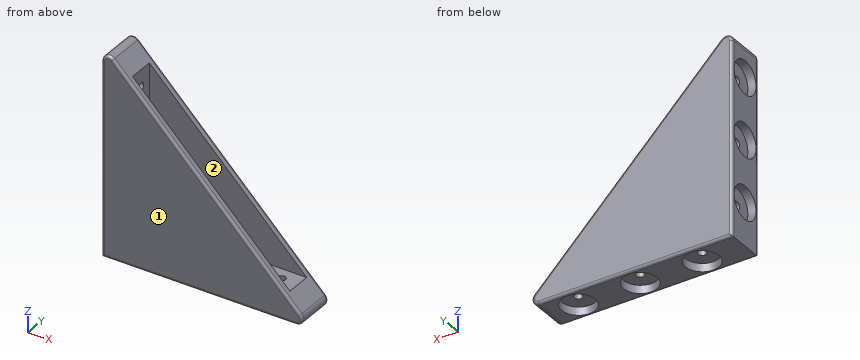
from build123d import *

# Parameters (mm, degrees)
F1_DEPTH  = 7.5
F2_R      = 6.375
F3_DEPTH  = 3.125
F4_R      = 6.375
F5_DEPTH  = 3.125
F6_W      = 60.104076
F6_H      = 60.104076
F7_DEPTH  = 4.875
F8_R      = 1.55
F9_DEPTH  = 76.876
F10_R     = 1.55
F11_DEPTH = 76.876
F12_R     = 2.5
F13_R     = 1


with BuildPart() as f1:
    # F0 (on Front) → F1 (new body, symmetric)
    with BuildSketch(Plane.XZ):
        Polygon((80, 0), (0, 80), (0, 0), align=None)
    extrude(amount=F1_DEPTH, both=True)

    # F2 (on face) → F3 (cut)
    with BuildSketch(Plane(origin=(0, 0, 0), x_dir=(0, -1, 0), z_dir=(-1, 0, 0))):
        with Locations((0, 63.625)):
            Circle(F2_R)
        with Locations((0, 40)):
            Circle(F2_R)
        with Locations((0, 16.375)):
            Circle(F2_R)
    extrude(amount=-F3_DEPTH, mode=Mode.SUBTRACT)

    # F4 (on face) → F5 (cut)
    with BuildSketch(Plane(origin=(0, 0, 0), x_dir=(1, 0, 0), z_dir=(0, 0, -1))):
        with Locations((16.375, 0)):
            Circle(F4_R)
        with Locations((40, 0)):
            Circle(F4_R)
        with Locations((63.625, 0)):
            Circle(F4_R)
    extrude(amount=-F5_DEPTH, mode=Mode.SUBTRACT)

    # F6 (on Front) → F7 (cut, symmetric)
    with BuildSketch(Plane.XZ):
        with Locations((40, 40)):
            Rectangle(F6_W, F6_H)
    extrude(amount=F7_DEPTH, both=True, mode=Mode.SUBTRACT)

    # F8 (on face) → F9 (cut, through all)
    with BuildSketch(Plane(origin=(3.125, 0, 0), x_dir=(0, -1, 0), z_dir=(-1, 0, 0))):
        with Locations((0, 63.625)):
            Circle(F8_R)
        with Locations((0, 40)):
            Circle(F8_R)
        with Locations((0, 16.375)):
            Circle(F8_R)
    extrude(amount=-F9_DEPTH, mode=Mode.SUBTRACT)

    # F10 (on face) → F11 (cut, through all)
    with BuildSketch(Plane(origin=(0, 0, 3.125), x_dir=(1, 0, 0), z_dir=(0, 0, -1))):
        with Locations((16.375, 0)):
            Circle(F10_R)
        with Locations((40, 0)):
            Circle(F10_R)
        with Locations((63.625, 0)):
            Circle(F10_R)
    extrude(amount=-F11_DEPTH, mode=Mode.SUBTRACT)

    # F12
    f12_edges = [f1.edges().sort_by_distance(p)[0] for p in [
        (0, 0, 80),
        (80, 0, 0),
    ]]
    fillet(f12_edges, radius=F12_R)

    # F13
    f13_edges = [f1.edges().sort_by_distance(p)[0] for p in [
        (40, -7.5, 40),
        (40, 7.5, 40),
    ]]
    fillet(f13_edges, radius=F13_R)


solid = f1.part
Check sheet for the modelled part. Datum: model origin and axes. Units: mm. Face numbers are marked on the shaded views. A direction names the side the tool comes from. Round coordinates to 2 decimals unless told otherwise and drop trailing zeros. One line per item, written item: value.
(1) Sectioned sample at B-B, the plane y = 0. Count the separate pieces of the cut face and the enclosed holes in it, then the cut area to 3 significant figures.
Computed values:
separate pieces: 7
enclosed holes: 0
area: 1,010 mm^2
(2) Access from +Z, -Z, +X, -X, +Y, -Y to the whole of each face (thin tool, end or side, straight path). Record for the marked faces 1 and 2.
Computed values:
face 1: +Z, -Z, +X, -X, -Y
face 2: +Z, +X
(3) Thickness scan on line 1 (Z direction, x = 2.3, y = 0) (3 decimals); line 2 (Y direction, x = 26, z = 43) (3 decimals); line 3 (X direction, y = 0, z = 6.5) (3 decimals). Record the ranges inside material, lowest first.
Computed values:
line 1: z = 0 to 10, 22.75 to 33.625, 46.375 to 57.25, 70 to 76.456
line 2: y = -7.5 to -4.875, 4.875 to 7.5
line 3: x = 0 to 14.825, 17.925 to 38.45, 41.55 to 62.075, 65.175 to 73.5
(4) Depth check by flat-ended pin: pin 1 Ø1.5 at (y, z) = (0, 42.5) entering from -X (3 decimals); pin 2 Ø3 at (y, z) = (-1, 49) entering from +X; pin 3 Ø3 at (y, z) = (0, 40) entering from +X; pin 4 Ø6 at (y, z) = (-6, 67) entering from +X. Enter the tip coordinate at first touch or a pass-through.
Computed values:
pin 1: stops at x = 3.125
pin 2: stops at x = 9.95
pin 3: passes through
pin 4: stops at x = 16
